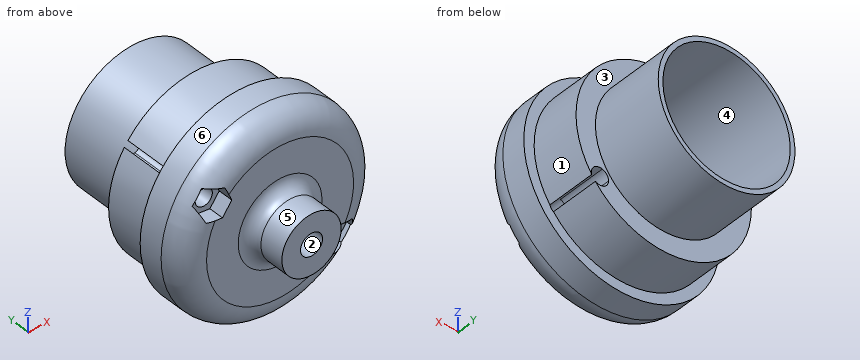
```python
from build123d import *

# Parameters (mm, degrees)
SKETCH1_R               = 17.9
SKETCH1_R_2             = 14.9
BOSS_EXTRUDE1_DEPTH     = 10
SKETCH2_R               = 20
BOSS_EXTRUDE2_DEPTH     = 10
FILLET1_R               = 5
SKETCH3_R               = 1.75
CUT_EXTRUDE1_DEPTH      = 1
CUT_EXTRUDE1_DEPTH_BACK = 332.06387935
CUT_EXTRUDE3_DEPTH      = 3
SKETCH8_R               = 13
BOSS_EXTRUDE3_DEPTH     = 10
SKETCH9_R               = 6.05
BOSS_EXTRUDE4_DEPTH     = 7.5
FILLET2_R               = 2.5
SKETCH11_R              = 2.25
CUT_EXTRUDE4_DEPTH      = 17.5
CUT_EXTRUDE5_DEPTH      = 3.5
SKETCH13_R              = 13.95
SKETCH13_R_2            = 13
BOSS_EXTRUDE5_DEPTH     = 15


with BuildPart() as part:
    # Sketch1 → Boss-Extrude1 (new body)
    with BuildSketch(Plane(origin=(0, -62.195205507, 0), x_dir=(-1, 0, 0), z_dir=(0, -1, 0))):
        with Locations((-0.536002938, -73.600816835)):
            Circle(SKETCH1_R)
        with Locations((-0.536002938, -73.600816835)):
            Circle(SKETCH1_R_2, mode=Mode.SUBTRACT)
    extrude(amount=BOSS_EXTRUDE1_DEPTH)

    # Sketch2 → Boss-Extrude2 (add)
    with BuildSketch(Plane(origin=(0, -72.195205507, 0), x_dir=(-1, 0, 0), z_dir=(0, -1, 0))):
        with Locations((-0.536002938, -73.600816835)):
            Circle(SKETCH2_R)
    extrude(amount=BOSS_EXTRUDE2_DEPTH)

    # Fillet1
    fillet1_edges = [part.edges().sort_by_distance(p)[0] for p in [
        (20.536002938, -82.195205507, 73.600816835),
    ]]
    fillet(fillet1_edges, radius=FILLET1_R)

    # Sketch3 → Cut-Extrude1 (cut, two sides)
    with BuildSketch(Plane(origin=(0, 248.868673843, 0), x_dir=(1, 0, 0), z_dir=(0, 1, 0))) as cut_extrude1_sk:
        with Locations((-12.468535925, -83.344762082)):
            Circle(SKETCH3_R)
        with Locations((13.5405418, -63.856871588)):
            Circle(SKETCH3_R)
    extrude(amount=CUT_EXTRUDE1_DEPTH, mode=Mode.SUBTRACT)
    extrude(cut_extrude1_sk.sketch, amount=-CUT_EXTRUDE1_DEPTH_BACK, mode=Mode.SUBTRACT)

    # Sketch7 → Cut-Extrude3 (cut)
    with BuildSketch(Plane(origin=(0, -82.195205507, 0), x_dir=(-1, 0, 0), z_dir=(0, -1, 0))):
        Polygon((10.564463201, -85.88599021), (13.717267678, -86.264351495), (15.621340402, -83.723123368), (14.372608649, -80.803533955), (11.219804171, -80.425172669), (9.315731448, -82.966400796), align=None)
        Polygon((-15.444614524, -66.398099716), (-12.291810047, -66.776461002), (-10.387737323, -64.235232874), (-11.636469076, -61.315643461), (-14.789273554, -60.937282175), (-16.693346277, -63.478510303), align=None)
    extrude(amount=-CUT_EXTRUDE3_DEPTH, mode=Mode.SUBTRACT)

    # Sketch8 → Boss-Extrude3 (add)
    with BuildSketch(Plane(origin=(0, -62.195205507, 0), x_dir=(1, 0, 0), z_dir=(0, 1, 0))):
        with BuildLine():
            ThreePointArc((16.682247488, -73.600816835), (16.107712715, -69.331968315), (14.424995948, -65.36691823))
            ThreePointArc((14.424995948, -65.36691823), (12.661441741, -65.370041468), (11.790660849, -63.836459442))
            ThreePointArc((11.790660849, -63.836459442), (-8.398445319, -61.676655048), (-11.996595259, -81.659599773))
            ThreePointArc((-11.996595259, -81.659599773), (-11.074190888, -82.287264131), (-10.718535925, -83.344762082))
            ThreePointArc((-10.718535925, -83.344762082), (-10.861687777, -84.037971309), (-11.267723389, -84.617770038))
            ThreePointArc((-11.267723389, -84.617770038), (6.456955614, -88.622252601), (16.682247488, -73.600816835))
        make_face()
        with Locations((0.536002938, -73.600816835)):
            Circle(SKETCH8_R, mode=Mode.SUBTRACT)
    extrude(amount=-BOSS_EXTRUDE3_DEPTH)

    # Sketch9 → Boss-Extrude4 (add)
    with BuildSketch(Plane.XZ.offset(82.195205507)):
        with Locations((0.536002938, 73.600816835)):
            Circle(SKETCH9_R)
    extrude(amount=BOSS_EXTRUDE4_DEPTH)

    # Fillet2
    fillet2_edges = [part.edges().sort_by_distance(p)[0] for p in [
        (-5.513997062, -82.195205507, 73.600816835),
    ]]
    fillet(fillet2_edges, radius=FILLET2_R)

    # Sketch11 → Cut-Extrude4 (cut)
    with BuildSketch(Plane(origin=(0, -89.695205507, 0), x_dir=(-1, 0, 0), z_dir=(0, -1, 0))):
        with Locations((-0.536002938, -73.600816835)):
            Circle(SKETCH11_R)
    extrude(amount=-CUT_EXTRUDE4_DEPTH, mode=Mode.SUBTRACT)

    # Sketch12 → Cut-Extrude5 (cut)
    with BuildSketch(Plane(origin=(0, -72.195205507, 0), x_dir=(1, 0, 0), z_dir=(0, 1, 0))):
        Polygon((2.981769599, -76.818200675), (4.545222407, -73.091412695), (2.099455746, -69.874028855), (-1.909763723, -70.383432996), (-3.473216532, -74.110220976), (-1.027449871, -77.327604816), align=None)
    extrude(amount=-CUT_EXTRUDE5_DEPTH, mode=Mode.SUBTRACT)

    # Sketch13 → Boss-Extrude5 (add)
    with BuildSketch(Plane(origin=(0, -62.195205507, 0), x_dir=(1, 0, 0), z_dir=(0, 1, 0))):
        with Locations((0.536002938, -73.600816835)):
            Circle(SKETCH13_R)
        with Locations((0.536002938, -73.600816835)):
            Circle(SKETCH13_R_2, mode=Mode.SUBTRACT)
    extrude(amount=BOSS_EXTRUDE5_DEPTH)


solid = part.part
```
Design review of the part built by this model. Coordinates are the model's own, in mm. Face numbers are marked on the shaded views. A direction names the side the tool comes from. Round coordinates to 2 decimals unless told otherwise and drop trailing zeros. Write each loop counter-clockwise with the first axis right and the second up, starting at its lowest first coordinate (ties: lowest second). Pieces come first, ordered by that corner, then holes. Notation, with made-up numbers: (3, 18) -> (11, 18) arc R19 ccw to (11, 54) -> close; hole circle Ø2 at (72.25, -2). An arc over 180 degrees is marked (long way). Write item = value, one per line. Start each with the question number.
1) Mouldability with a two-part tool opening along Z and no side actions: class the marked faces 1, 2 and 3 as +Z half, -Z half, draft (parallel to the pull), parting line (faces both ways), or undercut.
2) Wall thickness on probe 1 along Y at (x, z) = (-10, 75); probe 2 along X at (y, z) = (-65, 73.5); probe 3 along Z at (x, y) = (-7, -55): over which ranges is each line inside the solid? List them lowest first. Write a range as from..to.
3) Take a section at B-B, the plane y = -57. State the section outline as (x, z) points.
4) Tool access review of the marked faces 4, 5 and 6: name each direction out of +Z, -Z, +X, -X, +Y, -Y from which nothing blocks a thin tool from reaching the whole face with its end or side.
5) Clearance check with flat-ended pins moving along their axes: pin 1 (2 mm diameter, centred on x = 14, z = 65.5, fed in from -Y); pin 2 (8 mm diameter, centred on x = 5, z = 69.5, fed in from +Y); pin 3 (10 mm diameter, centred on x = 8, z = 59.5, fed in from -Y); pin 4 (2 mm diameter, centred on x = 13.54, z = 63.86, fed in from +Y). State where each tip first meets the part, or that it passes through.
Results list:
q1.face_1 = parting line
q1.face_2 = undercut
q1.face_3 = draft
q2.probe_1 = -82.2..-72.2
q2.probe_2 = -17.36..-12.46, 13.54..18.44
q2.probe_3 = 61.86..63.01, 84.19..85.34
q3.outline = circle Ø27.9 at (0.54, 73.6); hole circle Ø26 at (0.54, 73.6)
q4.face_4 = +Y
q4.face_5 = -Y
q4.face_6 = +Y, -Y
q5.pin_1 = -79.2
q5.pin_2 = -72.2
q5.pin_3 = -82.2
q5.pin_4 = through
